Geometry: final body of the model. Coordinates: model frame, mm. Give positions to 0.01 mm unless a question says otherwise; leave off trailing zeros. Write each loop counter-clockwise with the first axis right and the second up, starting at its lowest first coordinate (ties: lowest second). Pieces come first, ordered by that corner, then holes. Notation, with made-up numbers: (-13.5, 5.25) - (12.5, 5.25) arc R18 ccw to (12.5, 19.25) - close; hole circle Ø11 at (41, -6). An arc over 180 degrees is marked (long way). Use CSV: the item, a comma, the result in double quotes. Start each with the question number.
(1) Section B-B on y = 1.3. Output: boundary loops of the cut face in (x, z), and give its area (3 significant figures).
(2) Section A-A on x = 0. Output: boundary loops of the cut face in (y, z).
(3) Draft query along X for faces 1 (the cylindrical face through (1.802, 1.014, 5.723)), 2 (the flat face through (-1, 2, 14)). Return one class per face: released by +X, released by -X, zero draft, split by the parting line, or undercut.
(4) Line query: probe 1 along X at (y, z) = (1.45, 54.68); probe 2 along X at (y, z) = (0.6, 0); probe 3 along Z at (x, y) = (1.5, 1.95). Output: solid intervals per line, ascending. Write a range as [from, to].
(5) Section D-D on x = 25. Output: boundary loops of the cut face in (y, z), and give its area (3 significant figures).
(6) Section C-C on z = -36.5. Output: boundary loops of the cut face in (x, y), and give its area (3 significant figures).
from build123d import *

# Parameters (mm, degrees)
SKETCH1_R           = 50
BOSS_EXTRUDE1_DEPTH = 2
SKETCH2_R           = 6
CUT_EXTRUDE1_DEPTH  = 2
SKETCH3_W           = 36.555538841
SKETCH3_H           = 76.419948839
BOSS_EXTRUDE2_DEPTH = 2
CUT_EXTRUDE2_REACH  = 93.346
SKETCH8_R           = 1


with BuildPart() as part:
    # Sketch1 → Boss-Extrude1 (new body)
    with BuildSketch(Plane(origin=(0, 0, 0), x_dir=(1, 0, 0), z_dir=(0, 1, 0))):
        with Locations(Location((0, 0, 0), (0, 0, 270))):
            Circle(SKETCH1_R)
    extrude(amount=BOSS_EXTRUDE1_DEPTH)

    # Sketch2 → Cut-Extrude1 (cut)
    with BuildSketch(Plane(origin=(0, 2, 0), x_dir=(1, 0, 0), z_dir=(0, 1, 0))):
        with Locations(Location((0, 0, 0), (0, 0, 270))):
            Circle(SKETCH2_R)
    extrude(amount=-CUT_EXTRUDE1_DEPTH, mode=Mode.SUBTRACT)

    # Sketch3 → Boss-Extrude2 (add, through all)
    with BuildSketch(Plane.XZ):
        with Locations((-31.722230579, 38.209974419)):
            Rectangle(SKETCH3_W, SKETCH3_H)
    extrude(amount=-BOSS_EXTRUDE2_DEPTH)

    # Sketch8 → Cut-Extrude2 (cut, up to next)
    with BuildSketch(Plane.XZ, mode=Mode.PRIVATE) as cut_extrude2_sk1:
        with Locations(Location((-23.05, 54.68, 0), (0, 0, 270))):
            Circle(SKETCH8_R)
    cut_extrude2_tool1 = extrude(cut_extrude2_sk1.sketch, amount=-CUT_EXTRUDE2_REACH, mode=Mode.PRIVATE) & part.part
    add(cut_extrude2_tool1.solids().sort_by_distance((-23.05, 0, 54.68))[0], mode=Mode.SUBTRACT)


solid = part.part
Check values:
1,outline,"(-50, 0) arc R50 ccw (long way) to (-13.44, 48.16) - (-13.44, 76.42) - (-50, 76.42) - close; hole circle Ø2 at (-23.05, 54.68); hole circle Ø12 at (0, 0)"
1,area,"9,230 mm²"
2,outline,"(0, -50) - (2, -50) - (2, -6) - (0, -6) - close; (0, 6) - (2, 6) - (2, 50) - (0, 50) - close"
3,face 1,"undercut"
3,face 2,"zero draft"
4,probe 1,"x = [-50, -24.05], [-22.05, -13.44]"
4,probe 2,"x = [-50, -6], [6, 50]"
4,probe 3,"z = [-49.98, -5.81], [5.81, 49.98]"
5,outline,"(0, -43.3) - (2, -43.3) - (2, 43.3) - (0, 43.3) - close"
5,area,"173 mm²"
6,outline,"(-34.17, 0) - (34.17, 0) - (34.17, 2) - (-34.17, 2) - close"
6,area,"137 mm²"
